Autodesk Inventor part; units mm, degrees
ref_plane "YZ Plane" through (0, 0, 0) normal (1, 0, 0) x (0, 1, 0)
ref_plane "XZ Plane" through (0, 0, 0) normal (0, 1, 0) x (-1, 0, 0)
ref_plane "XY Plane" through (0, 0, 0) normal (0, 0, 1) x (1, 0, 0)
sketch "Sketch1" plane through (0, 0, 0) normal (0, 0, 1) x (1, 0, 0)
  line L0 (-58, -60) -> (-60, -60)
  line L1 (-60, -60) -> (-60, -39.5)
  line L2 (-60, -39.5) -> (-58, -39.5)
  line L3 (-58, -39.5) -> (-58, -60)
  line L4 (49.6, 30) -> (51.6, 30)
  line L5 (51.6, 30) -> (51.6, 9.5)
  line L6 (51.6, 9.5) -> (49.6, 9.5)
  line L7 (49.6, 9.5) -> (49.6, 30)
  line L8 (-58, 39.5) -> (-60, 39.5)
  line L9 (-60, 39.5) -> (-60, 60)
  line L10 (-60, 60) -> (-58, 60)
  line L11 (-58, 60) -> (-58, 39.5)
  line L12 (-21.6, -39.5) -> (-19.6, -39.5)
  line L13 (-19.6, -39.5) -> (-19.6, -60)
  line L14 (-19.6, -60) -> (-21.6, -60)
  line L15 (-21.6, -60) -> (-21.6, -39.5)
  line L16 (51.6, -30) -> (49.6, -30)
  line L17 (49.6, -30) -> (49.6, -9.5)
  line L18 (49.6, -9.5) -> (51.6, -9.5)
  line L19 (51.6, -9.5) -> (51.6, -30)
  line L20 (-21.6, 60) -> (-19.6, 60)
  line L21 (-19.6, 60) -> (-19.6, 39.5)
  line L22 (-19.6, 39.5) -> (-21.6, 39.5)
  line L23 (-21.6, 39.5) -> (-21.6, 60)
  line L24 (90, -35) -> (90, 35)
  line L25 (90, 35) -> (49.6, 35)
  line L26 (49.6, 35) -> (49.6, 60)
  line L27 (49.6, 60) -> (90, 60)
  line L28 (90, 60) -> (90, 90)
  line L29 (90, 90) -> (-19.6, 90)
  line L30 (-19.6, 90) -> (-19.6, 65)
  line L31 (-19.6, 65) -> (-60, 65)
  line L32 (-60, 65) -> (-60, 90)
  line L33 (-60, 90) -> (-90, 90)
  line L34 (-90, 90) -> (-90, -90)
  line L35 (-90, -90) -> (-60, -90)
  line L36 (-60, -90) -> (-60, -65)
  line L37 (-60, -65) -> (-19.6, -65)
  line L38 (-19.6, -65) -> (-19.6, -90)
  line L39 (-19.6, -90) -> (90, -90)
  line L40 (90, -90) -> (90, -60)
  line L41 (90, -60) -> (49.6, -60)
  line L42 (49.6, -60) -> (49.6, -35)
  line L43 (49.6, -35) -> (90, -35)
  line L44 (86, -32) -> (73.8, -32)
  line L45 (73.8, -32) -> (73.8, -7.5)
  line L46 (73.8, -7.5) -> (86, -7.5)
  line L47 (86, -7.5) -> (86, -32)
  line L48 (65.8, -32) -> (53.6, -32)
  line L49 (53.6, -32) -> (53.6, -7.5)
  line L50 (53.6, -7.5) -> (65.8, -7.5)
  line L51 (65.8, -7.5) -> (65.8, -32)
  line L52 (86, -86) -> (70.6, -86)
  line L53 (70.6, -86) -> (70.6, -69.8)
  line L54 (70.6, -69.8) -> (86, -69.8)
  line L55 (86, -69.8) -> (86, -86)
  line L56 (86, 86) -> (86, 69.8)
  line L57 (86, 69.8) -> (70.6, 69.8)
  line L58 (70.6, 69.8) -> (70.6, 86)
  line L59 (70.6, 86) -> (86, 86)
  line L60 (73.8, 32) -> (86, 32)
  line L61 (86, 32) -> (86, 7.5)
  line L62 (86, 7.5) -> (73.8, 7.5)
  line L63 (73.8, 7.5) -> (73.8, 32)
  line L64 (65.8, 32) -> (65.8, 7.5)
  line L65 (65.8, 7.5) -> (53.6, 7.5)
  line L66 (53.6, 7.5) -> (53.6, 32)
  line L67 (53.6, 32) -> (65.8, 32)
  line L68 (-69.6, -87) -> (-85, -87)
  line L69 (-85, -87) -> (-85, -70.8)
  line L70 (-85, -70.8) -> (-69.6, -70.8)
  line L71 (-69.6, -70.8) -> (-69.6, -87)
  line L72 (-56, -62) -> (-56, -37.5)
  line L73 (-56, -37.5) -> (-43.8, -37.5)
  line L74 (-43.8, -37.5) -> (-43.8, -62)
  line L75 (-43.8, -62) -> (-56, -62)
  line L76 (-56, 62) -> (-43.8, 62)
  line L77 (-43.8, 62) -> (-43.8, 37.5)
  line L78 (-43.8, 37.5) -> (-56, 37.5)
  line L79 (-56, 37.5) -> (-56, 62)
  line L80 (-23.6, 62) -> (-23.6, 37.5)
  line L81 (-23.6, 37.5) -> (-35.8, 37.5)
  line L82 (-35.8, 37.5) -> (-35.8, 62)
  line L83 (-35.8, 62) -> (-23.6, 62)
  line L84 (-23.6, -62) -> (-35.8, -62)
  line L85 (-35.8, -62) -> (-35.8, -37.5)
  line L86 (-35.8, -37.5) -> (-23.6, -37.5)
  line L87 (-23.6, -37.5) -> (-23.6, -62)
  line L88 (-85, 87) -> (-69.6, 87)
  line L89 (-69.6, 87) -> (-69.6, 70.8)
  line L90 (-69.6, 70.8) -> (-85, 70.8)
  line L91 (-85, 70.8) -> (-85, 87)
  circle A0 centre (87, -63) radius 2
  line L92 (90, -60) -> (90, -66)
  line L93 (84, -60) -> (90, -60)
  line L94 (84, -63) -> (84, -60)
  line L95 (90, -66) -> (87, -66)
  line L96 (-19.6, 68) -> (-16.6, 68)
  line L97 (-16.6, 68) -> (-16.6, 84)
  line L98 (-13.6, 87) -> (46.6, 87)
  line L99 (52.6, 87) -> (87, 87)
  line L100 (87, 87) -> (87, 66)
  line L101 (84, 63) -> (84, 60)
  line L102 (84, 60) -> (90, 60)
  line L103 (90, 60) -> (90, 90)
  line L104 (90, 90) -> (-19.6, 90)
  line L105 (-19.6, 90) -> (-19.6, 68)
  line L106 (90, -66) -> (87, -66)
  line L107 (87, -66) -> (87, -90)
  line L108 (87, -90) -> (90, -90)
  line L109 (90, -90) -> (90, -66)
  line L110 (87, -90) -> (-19.6, -90)
  line L111 (-19.6, -90) -> (-19.6, -87)
  line L112 (-19.6, -87) -> (87, -87)
  line L113 (87, -87) -> (87, -90)
  line L114 (-19.6, -87) -> (-16.6, -87)
  line L115 (-16.6, -87) -> (-16.6, -65)
  line L116 (-16.6, -65) -> (-19.6, -65)
  line L117 (-19.6, -65) -> (-19.6, -87)
  line L118 (-19.6, -65) -> (-16.6, -65)
  line L119 (-16.6, -65) -> (-16.6, -68)
  line L120 (-16.6, -68) -> (-19.6, -68)
  line L121 (-19.6, -68) -> (-19.6, -65)
  line L122 (-19.6, -68) -> (-13.6, -68)
  line L123 (-13.6, -68) -> (-13.6, -62)
  line L124 (-13.6, -62) -> (-19.6, -62)
  line L125 (-19.6, -62) -> (-19.6, -68)
  line L126 (-19.6, -90) -> (-13.6, -90)
  line L127 (-13.6, -90) -> (-13.6, -84)
  line L128 (-13.6, -84) -> (-19.6, -84)
  line L129 (-19.6, -84) -> (-19.6, -90)
  line L130 (46.6, -90) -> (52.6, -90)
  line L131 (52.6, -90) -> (52.6, -84)
  line L132 (52.6, -84) -> (46.6, -84)
  line L133 (46.6, -84) -> (46.6, -90)
  circle A1 centre (-63, -65) radius 1.5
  circle A2 centre (-16.6, -87) radius 1.5
  circle A3 centre (49.6, -87) radius 1.5
  circle A4 centre (46.6, -60) radius 1.5
  circle A5 centre (87, -63) radius 1.5
  circle A6 centre (46.6, -32) radius 1.5
  circle A7 centre (46.6, 32) radius 1.5
  circle A8 centre (87, 63) radius 1.5
  circle A9 centre (46.6, 60) radius 1.5
  circle A10 centre (49.6, 87) radius 1.5
  circle A11 centre (-16.6, 87) radius 1.5
  circle A12 centre (-16.6, 65) radius 1.5
  circle A13 centre (-63, 65) radius 1.5
  arc A14 (87, 66) -> (84, 63) centre (87, 63) ccw
  arc A15 (-16.6, 84) -> (-13.6, 87) centre (-16.6, 87) ccw
  arc A16 (46.6, 87) -> (52.6, 87) centre (49.6, 87) ccw
  arc A17 (84, -63) -> (87, -66) centre (87, -63) ccw
  line L134 (-76, -39.25) -> (-82, -39.25)
  line L135 (-82, -39.25) -> (-82, -20.75)
  line L136 (-82, -20.75) -> (-76, -20.75)
  line L137 (-76, -20.75) -> (-76, -39.25)
  line L138 (-76, 20.75) -> (-82, 20.75)
  line L139 (-82, 20.75) -> (-82, 39.25)
  line L140 (-82, 39.25) -> (-76, 39.25)
  line L141 (-76, 39.25) -> (-76, 20.75)
  circle A18 centre (-87, 55.8) radius 1.25
  circle A19 centre (-87, -55.8) radius 1.25
  point P0 (0, 0)
  point P1 (52.6, -87)
  point P2 (46.6, -87)
  point P3 (-13.6, -87)
  point P4 (-16.6, -84)
  dimension "d0" = 3
  dimension "d1" = 3
  dimension "d2" = 6
  dimension "d3" = 6
  dimension "d4" = 6
  dimension "d5" = 6
  dimension "d6" = 6
  dimension "d7" = 6
extrude "Extrusion1" add sketch "Sketch1" along normal blind 8 contours L41 L40 L95 A17 L94 | L40 L39 L107 L95 | L107 L39 L131 L112 | L131 L39 L133 L112 A3 | L112 A3 L133 L132 L131 | A3 L112 | L112 A3 | L39 L127 L112 L133 | L39 L38 L112 A2 L127 | L112 A2 L115 L128 L127 | L38 L128 L115 A2 L112 | A2 L112 | L112 L115 A2 | L38 L120 L115 L128 | A2 L115 L112 | L38 L116 L115 L120 | L115 L116 L125 L124 L123 L122 | A0 | A5
sketch "Sketch2" plane through (0, 0, 0) normal (0, 0, -1) x (-1, 0, 0)
  line L0 (-84, -66) -> (-87, -66)
  line L1 (-90, -90) -> (-90, -60)
  line L2 (-84, -66) -> (-90, -66)
  line L3 (-90, -66) -> (-90, -60)
  line L4 (-90, -60) -> (-84, -60)
  line L5 (-84, -60) -> (-84, -66)
  line L6 (-84, -60) -> (-90, -66)
  line L7 (-90, -60) -> (-84, -66)
  circle A0 centre (-87, -63) radius 2
  line L8 (-52.6, -84) -> (-46.6, -84)
  line L9 (-46.6, -84) -> (-52.6, -90)
  line L10 (19.6, -90) -> (-90, -90)
  line L11 (-52.6, -84) -> (-46.6, -90)
  line L12 (-46.6, -90) -> (-46.6, -84)
  line L13 (-52.6, -84) -> (-52.6, -90)
  circle A1 centre (-49.6, -87) radius 2
  line L14 (13.6, -84) -> (16.6, -84)
  line L15 (13.6, -84) -> (19.6, -90)
  line L16 (19.6, -62) -> (19.6, -90)
  line L17 (19.6, -84) -> (13.6, -90)
  line L18 (19.6, -84) -> (13.6, -84)
  circle A2 centre (16.6, -87) radius 2
  line L19 (13.6, -68) -> (13.6, -62)
  line L20 (13.6, -68) -> (19.6, -62)
  line L21 (19.6, -68) -> (13.6, -62)
  line L22 (13.6, -62) -> (13.6, -68)
  line L23 (19.6, -68) -> (13.6, -68)
  circle A3 centre (16.6, -65) radius 2
  point P0 (0, 0)
  point P1 (19.6, -87)
  dimension "d10" = 4
  dimension "d11" = 4
  dimension "d12" = 4
  dimension "d13" = 4
extrude "Extrusion2" cut sketch "Sketch2" against normal blind 6 contours A1 L9 L11 | L11 L9 A1 | A1 L11 L9 | L11 A1 L9 | A2 L17 L15 | L15 L17 A2 | A2 L15 L17 | L15 A2 L17
extrude "Extrusion3" cut sketch "Sketch2" against normal blind 7 contours A0 L6 L7 | L7 L6 A0 | L6 L7 A0 | L6 A0 L7
extrude "Extrusion4" cut sketch "Sketch2" against normal blind 3 contours L7 A0 L6 L5 | L0 L2 L6 A0 L7 | L6 A0 L7 L4 | L1 L7 A0 L6
sketch "Sketch3" plane through (0, 0, 8) normal (0, 0, 1) x (1, 0, 0)
  line L0 (-16.6, -68) -> (-13.6, -68)
  line L1 (-19.6, -62) -> (-19.6, -90)
  line L2 (-13.6, -68) -> (-19.6, -62)
  line L3 (-19.6, -62) -> (-13.6, -62)
  line L4 (-13.6, -62) -> (-19.6, -68)
  line L5 (-13.6, -68) -> (-19.6, -68)
  line L6 (-13.6, -62) -> (-13.6, -68)
  circle A0 centre (-16.6, -65) radius 1.65
  point P0 (0, 0)
  point P1 (-19.6, -87)
  point P2 (-17.7667, -66.1667)
  point P3 (-17.7667, -63.8333)
  dimension "d20" = 3.3
extrude "Extrusion5" cut sketch "Sketch3" against normal blind 5 contours L5 L4 A0 L2 L0 | L2 A0 L4 L6 | L1 L2 A0 L4 | L4 A0 L2 L3
extrude "Extrusion6" cut sketch "Sketch3" against normal blind 8 contours A0 L4 L2 | L2 L4 A0 | A0 L2 L4 | L2 A0 L4
fillet "Fillet1" radius 3 5 edges at (52.6, -84, 4) (46.6, -84, 4) (-13.6, -68, 1.5) (-13.6, -62, 1.5) (-13.6, -84, 4)
properties part number "rightwall2"
CAD build for the part. Positions are in the model's coordinates, mm. A direction names the side the tool comes from. Give positions to 0.01 mm unless a question says otherwise; leave off trailing zeros. Order: outer loops, then holes, each group sorted by start corner. A loop starts at its lowest first (then second) coordinate and runs counter-clockwise, first axis right, second up.
(1) Flat gauge pins, fed straight in: pin 1 (3.5 mm diameter, centred on x = -18.5, z = 1.5, fed in from +Y); pin 2 (4.5 mm diameter, centred on x = 87.5, y = -63.5, fed in from -Z); pin 3 (1.2 mm diameter, centred on x = -17, y = -88, fed in from -Z); pin 4 (1.2 mm diameter, centred on x = 48.5, y = -88, fed in from -Z). Where does each tip first touch, or does it go through?
(2) Saw through at B-B, the plane y = -73.75. Give the cut face in (x, z), then the cut area to 3 significant figures.
(3) Saw through at A-A, the plane z = 1.25. State how many separate pieces and enclosed holes the cut face has, then the cut area to 3 significant figures.
(4) Drill centre lines: L1, parallel to Y at x = 49.6, z = 3.6; L2, parallel to X at y = -80, z = 0.5; L3, parallel to X at y = -65, z = 1.1. Where is each one in solid material? Low to high.
(5) Saw through at C-C, the plane x = 17. Give the cut face in (y, z), then the cut area to 3 significant figures.
(6) Tool access for faces 5 (the flat face through (-17, -87, 6)), 6 (the flat face through (88, -66, 1)), 7 (the flat face through (16, -87, 4)): list every direction of +Z, -Z, +X, -X, +Y, -Y with a clear straight run to the whole face (end or side of a thin tool).
(7) Mould opens along X. For faces 1 (the cylindrical face through (-15.839, -66.464, 1.521)), 2 (the flat face through (84, -62, 5)), 3 (the flat face through (-18, -62, 1)), 4 (the cylindrical face through (51.74, -84.9, 4.06)) say: released by +X, released by -X, zero draft, split by the parting line, or undercut.
Results found:
1. pin 1: stops at y = -62
1. pin 2: stops at z = 3
1. pin 3: stops at z = 6
1. pin 4: stops at z = 0
2. outline: (-19.6, 0) - (-16.6, 0) - (-16.6, 8) - (-19.6, 8) - close; (87, 0) - (90, 0) - (90, 8) - (87, 8) - close
2. area: 48.0 mm2
3. separate pieces: 1
3. enclosed holes: 3
3. area: 468 mm2
4. L1: y = -90 to -89, -85 to -84
4. L2: x = -19.6 to -16.6, 87 to 90
4. L3: x = -19.6 to -18.25, -14.95 to -13.6
5. outline: (-90, 0) - (-87, 0) - (-87, 8) - (-90, 8) - close
5. area: 24.0 mm2
6. face 5: -Z
6. face 6: -Z, +X, +Y
6. face 7: +Z, -Z, +Y
7. face 1: undercut
7. face 2: released by -X
7. face 3: zero draft
7. face 4: undercut
